from build123d import *

# Parameters (mm, degrees)
CASE_SKETCH_W        = 19.8
CASE_SKETCH_H        = 10.2
CASE_2_DEPTH         = 6.4
SCREW_HOLES_SKETCH_R = 1.1
SCREW_HOLES_DEPTH    = 30
PLUNGER_SKETCH_W     = 2.5
PLUNGER_SKETCH_H     = 0.7
PLUNGER_DEPTH        = 2.5


with BuildPart() as part:
    # Case Sketch → Case 2 (new body)
    with BuildSketch(Plane.XY.offset(13.6)):
        with Locations((-856.1, 155.6)):
            Rectangle(CASE_SKETCH_W, CASE_SKETCH_H)
    extrude(amount=CASE_2_DEPTH)

    # Screw Holes Sketch → Screw Holes (cut, symmetric)
    with BuildSketch(Plane.XY):
        with Locations((-860.75, 155.6)):
            Circle(SCREW_HOLES_SKETCH_R)
        with Locations((-851.25, 155.6)):
            Circle(SCREW_HOLES_SKETCH_R)
    extrude(amount=SCREW_HOLES_DEPTH, both=True, mode=Mode.SUBTRACT)

    # Plunger Sketch → Plunger (add)
    with BuildSketch(Plane.XY.offset(15.55)):
        with Locations((-848, 150.15)):
            Rectangle(PLUNGER_SKETCH_W, PLUNGER_SKETCH_H)
    extrude(amount=PLUNGER_DEPTH)


solid = part.part
Read the model definition and answer for the solid it produces. Units are mm, in the model's axes. Round coordinates to 2 decimals unless told otherwise and drop trailing zeros. Order: outer loops, then holes, each group sorted by start corner. A loop starts at its lowest first (then second) coordinate and runs counter-clockwise, first axis right, second up.
1) The part is cut by section D-D on z = 15. Write down the section's boundary in (x, y), plus the area to 3 significant figures.
2) The part is cut by section A-A on y = 155.6. Write down the section's boundary in (x, z).
3) The part is cut by section C-C on x = -860.75. Write down the section's boundary in (y, z), plus the area to 3 significant figures.
4) Flat-ended cylindrical pins translate along their axes: pin 1 (3 mm diameter, centred on x = -860.75, y = 155.6, fed in from -Z); pin 2 (0.8 mm diameter, centred on y = 150, z = 17, fed in from -X). Find the tip coordinate at first contact, or state that the pin passes through.
5) Straight lines are drawn through the part: L1, parallel to X at y = 155.6, z = 17; L2, parallel to Y at x = -860.75, z = 15.75; L3, parallel to Y at x = -852.5, z = 16.5. For each, find the intervals that lie inside material, in ascending order.
6) The part is cut by section B-B on z = 17.5. Write down the section's boundary in (x, y), plus the area to 3 significant figures.
7) The mould has two halves that part along Y. Classify faces 1 (the face through (-856, 160.7, 17)), 2 (the face through (-850.2, 155.93, 16.84)), 3 (the face through (-856, 156, 13.6)), 4 (the face through (-859.7, 155.93, 16.76)): released by +Y, released by -Y, zero draft, split by the parting line, or undercut.
Resolved:
1. outline: (-866, 150.5) - (-846.2, 150.5) - (-846.2, 160.7) - (-866, 160.7) - close; hole circle Ø2.2 at (-860.75, 155.6); hole circle Ø2.2 at (-851.25, 155.6)
1. area: 194 mm2
2. outline: (-866, 13.6) - (-861.85, 13.6) - (-861.85, 20) - (-866, 20) - close; (-859.65, 13.6) - (-852.35, 13.6) - (-852.35, 20) - (-859.65, 20) - close; (-850.15, 13.6) - (-846.2, 13.6) - (-846.2, 20) - (-850.15, 20) - close
3. outline: (150.5, 13.6) - (154.5, 13.6) - (154.5, 20) - (150.5, 20) - close; (156.7, 13.6) - (160.7, 13.6) - (160.7, 20) - (156.7, 20) - close
3. area: 51.2 mm2
4. pin 1: stops at z = 13.6
4. pin 2: stops at x = -849.25
5. L1: x = -866 to -861.85, -859.65 to -852.35, -850.15 to -846.2
5. L2: y = 150.5 to 154.5, 156.7 to 160.7
5. L3: y = 150.5 to 160.7
6. outline: (-866, 150.5) - (-849.25, 150.5) - (-849.25, 149.8) - (-846.75, 149.8) - (-846.75, 150.5) - (-846.2, 150.5) - (-846.2, 160.7) - (-866, 160.7) - close; hole circle Ø2.2 at (-860.75, 155.6); hole circle Ø2.2 at (-851.25, 155.6)
6. area: 196 mm2
7. face 1: released by +Y
7. face 2: undercut
7. face 3: zero draft
7. face 4: undercut
